Autodesk Inventor part; units mm, degrees
ref_plane "Work Plane1" through (2.75, 0, 0) normal (0, -1, 0) x (1, 0, 0)
ref_plane "YZ Plane" through (0, 0, 0) normal (1, 0, 0) x (0, 1, 0)
ref_plane "XZ Plane" through (0, 0, 0) normal (0, 1, 0) x (-1, 0, 0)
sketch "Skizze1" plane through (0, 0, 0) normal (0, 0, 1) x (1, 0, 0)
  line L0 (40, 6) -> (40, 0)
  line L1 (-18, 0) -> (40, 0)
  line L2 (-29.6, 0) -> (51.6, 0)
  line L3 (0, 7.2) -> (0, -1.2)
  line L4 (-18, 6) -> (-18, 0)
  line L5 (10, 6) -> (10, 0) construction
  line L6 (-29.6, 0) -> (51.6, 0)
  line L7 (-18, 6) -> (40, 6)
  dimension "d4" = 18
  dimension "d5" = 40
  dimension "d6" = 30
  dimension "d13" = 12
revolve "Körper" add sketch "Skizze1" angle 360 about axis through (-18, 0, 0) along (1, 0, 0)
thread "Gewinde1"
thread "Gewinde2"
chamfer "Fase1" distance 0.7678 distance2 0.7668 1 edges at (40, -6, 0) measured on face at (40, -3.0269, -1.5886)
chamfer "Fase2" distance 0.6776 distance2 0.7668 1 edges at (-18, -6, 0) measured on face at (20.1555, 5.9805, -0.4828)
ref_plane "Work Plane1" through (2.75, 0, 0) normal (0, -1, 0) x (1, 0, 0)
equation "\"d4\" = KOH"
equation "\"d5\" = NLG"
equation "\"d6\" = GEL"
equation "\"d13\" = GD"
equation "\"d1\" = KOH"
equation "\"d7\" = GEL + GAL"
equation "\"d10\" = -0.5 * SPD + 0.5 * GD"
equation "\"d12\" = -0.5 * SPD + 0.5 * GD"
equation "\"NLG\" = 40"
equation "\"GEL\" = 30"
equation "\"GAL\" = 0.61345 * PTC"
equation "\"SPD\" = NND - 1.2269 * PTC"
equation "\"d0\" = GD"
equation "\"GUL\" = 0.61345 * PTC"
equation "\"KOH\" = 18"
equation "\"GD\" = NND"
equation "\"BDM\" = NND"
equation "\"GUL1\" = 0.67658"
equation "\"GAL1\" = GAL"
equation "\"d80\" = -GUL - GEL"
equation "\"d86\" = -KOH + GUL1"
equation "\"PTC\" = 1.25"
equation "\"THREADDIA\" = 12"
equation "\"TOA\" = 30deg"
equation "\"NND\" = 12"
equation "\"GD1\" = THREADDIA - 1.2269 * PTC"
properties part number "UNI 5910 - M12 x 1,25 x 40" material "Steel, Mild"
Verification items for the finished model (mm, model axes). Coordinates: 2 decimals unless noted, no trailing zeros. Order: outer loops, then holes, each group sorted by start corner. A loop starts at its lowest first (then second) coordinate and runs counter-clockwise, first axis right, second up. Notation, with made-up numbers: (89, 80) - (123, 80) arc R5 cw to (123, 86) - close; hole circle Ø6 at (85.25, 33.25). An arc over 180 degrees is marked (long way). Return JSON: item names as keys, results as strings.
(1) Section check A-A, the plane x = 17. Record the cut outline in (y, z).
Filled sheet:
{"outline": "circle Ø12 at (0, 0)"}
(2) Go/stop test with flat-tipped pins: pin 1 (6 mm diameter, centred on x = -8.5, z = 4.5, fed in from -Y); pin 2 (3 mm diameter, centred on x = 4.5, y = -2, fed in from -Z); pin 3 (4 mm diameter, centred on x = -9.5, y = -4.5, fed in from -Z). Record where each tip stops, or that it passes through.
Filled sheet:
{"pin 1": "stops at y = -5.81", "pin 2": "stops at z = -5.98", "pin 3": "stops at z = -5.45"}
(3) Thickness scan on line 1 along Y through (x, z) = (-3.5, 0.25); line 2 along Y through (x, z) = (2.5, 4.25); line 3 along Z through (x, y) = (37, 3.75). Record the ranges inside material, lowest first.
Filled sheet:
{"line 1": "y = -5.99 to 5.99", "line 2": "y = -4.24 to 4.24", "line 3": "z = -4.68 to 4.68"}
